Work out the finished part from the listing and answer in its coordinate system (mm). Face numbers are marked on the shaded views. A direction names the side the tool comes from. Coordinates: 2 decimals unless noted, no trailing zeros. Order: outer loops, then holes, each group sorted by start corner. A loop starts at its lowest first (then second) coordinate and runs counter-clockwise, first axis right, second up. Notation, with made-up numbers: M 83.5,79 L 131.5,79 A21 ccw 131.5,106 Z; hole C 33.5,56.5 d3. An arc over 180 degrees is marked long. Answer in a Markdown table with one row per item. Add a question column.
Item 1: Which of the six approach directions +Z, -Z, +X, -X, +Y, -Y give full straight-line access (tool end or side, diameter ignored) to the marked faces 1, 2 and 3?
Item 2: The part is cut by section A-A (y = 55). Write down the section's boundary in (x, z), then the cut area to 3 significant figures.
Item 3: Consider line 1 (Y direction, x = -0.25, z = -1.5); line 2 (Y direction, x = -0.25, z = -4); line 3 (X direction, y = 31.5, z = -8). Determine where each line is inside the solid, lowest interval first. Write a range as from..to.
Item 4: Flat-ended cylindrical pins translate along their axes: pin 1 Ø4 at (x, z) = (1, -6.5) entering from +Y; pin 2 Ø1.7 at (y, z) = (16, -4) entering from +X; pin 3 Ø1.5 at (x, y) = (6, -31.5) entering from +Z. Find the tip coordinate at first contact, or state that the pin passes through.
Item 5: The part is cut by section B-B (z = -2). State how many separate pieces and enclosed holes the cut face has, then the cut area to 3 significant figures.
Item 6: The part is cut by section C-C (y = -76). Write down the section's boundary in (x, z), then the cut area to 3 significant figures.
Item 7: The mould has two halves that part along X. Classify the marked faces 4, 5 and 6: released by +X, released by -X, zero draft, split by the parting line, or undercut.
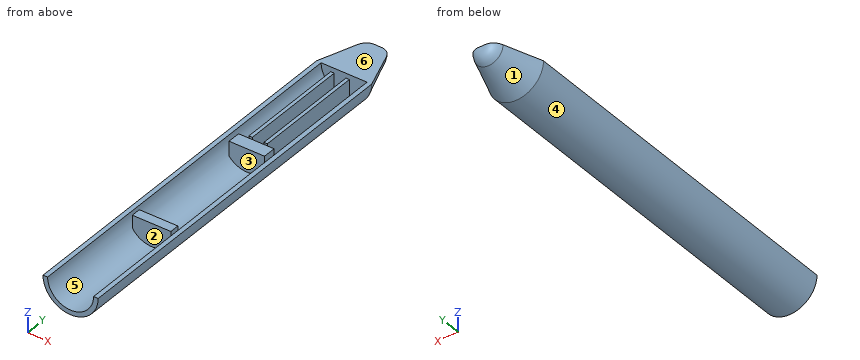
from build123d import *

# Parameters (mm, degrees)
SKETCH2_W                = 2
SKETCH2_H                = 162.039928857
BOSS_EXTRUDE1_REACH      = 94.669
BOSS_EXTRUDE1_END_RADIUS = 10
SKETCH4_W                = 15.457813272
SKETCH4_H                = 5.65259454
SKETCH4_W_2              = 16.763190872
SKETCH4_H_2              = 4.156828513
SKETCH4_W_3              = 1.5
SKETCH4_H_3              = 48.554461885
BOSS_EXTRUDE2_REACH      = 104.169
BOSS_EXTRUDE2_START      = -9.5
SKETCH4_4_W              = 5.08
SKETCH4_4_H              = 48.554461885
SKETCH5_W                = 72.783621468
SKETCH5_H                = 192.84631039
CUT_EXTRUDE1_DEPTH       = 93.66850023


with BuildPart() as part:
    # Sketch1 → Revolve1 (revolve)
    with BuildSketch(Plane.XY, mode=Mode.PRIVATE) as revolve1_sk:
        with BuildLine():
            Line((6.354000149, 87.279039692), (12, 71))
            Line((12, 71), (0, 71))
            Line((0, 71), (0, 91))
            add(Edge.make_bspline(
                [(0, 91), (4.668589185, 91.723642341), (6.354000149, 87.279039692)],
                knots=[0, 0, 0, 1, 1, 1], degree=2))
        make_face()
    revolve(revolve1_sk.sketch.rotate(Axis((0, 91, 0), (0, -1, 0)), 180), axis=Axis((0, 91, 0), (0, -1, 0)))

    # Sketch2 → Revolve2 (revolve)
    with BuildSketch(Plane.XY, mode=Mode.PRIVATE) as revolve2_sk:
        with Locations((11, -10.019964429)):
            Rectangle(SKETCH2_W, SKETCH2_H)
    revolve(revolve2_sk.sketch.rotate(Axis((0, 91, 0), (0, -1, 0)), 180), axis=Axis((0, 91, 0), (0, -1, 0)))

    # Boss-Extrude1: up to this cylinder (the profile starts inside it)
    boss_extrude1_end = Plane(origin=(0, 1.68519, 0), z_dir=(0, 1, 0)) * Cylinder(BOSS_EXTRUDE1_END_RADIUS, 295.657228, mode=Mode.PRIVATE)
    # Sketch4 → Boss-Extrude1 (add, up to the surface)
    with BuildSketch(Plane.XY, mode=Mode.PRIVATE) as boss_extrude1_sk1:
        with Locations((0, 16.17370273)):
            Rectangle(SKETCH4_W, SKETCH4_H)
    boss_extrude1_tool1 = extrude(boss_extrude1_sk1.sketch, amount=-BOSS_EXTRUDE1_REACH, mode=Mode.PRIVATE) & boss_extrude1_end
    add(boss_extrude1_tool1.solids().sort_by_distance((0, 16.173703, 0))[0])
    # Sketch4 → Boss-Extrude1 (add, up to the surface)
    with BuildSketch(Plane.XY, mode=Mode.PRIVATE) as boss_extrude1_sk2:
        with Locations((0, -40.974423961)):
            Rectangle(SKETCH4_W_2, SKETCH4_H_2)
    boss_extrude1_tool2 = extrude(boss_extrude1_sk2.sketch, amount=-BOSS_EXTRUDE1_REACH, mode=Mode.PRIVATE) & boss_extrude1_end
    add(boss_extrude1_tool2.solids().sort_by_distance((0, -40.974424, 0))[0])
    # Sketch4 → Boss-Extrude1 (add, up to the surface)
    with BuildSketch(Plane.XY, mode=Mode.PRIVATE) as boss_extrude1_sk3:
        with Locations((3.29, 44.344804049)):
            Rectangle(SKETCH4_W_3, SKETCH4_H_3)
    boss_extrude1_tool3 = extrude(boss_extrude1_sk3.sketch, amount=-BOSS_EXTRUDE1_REACH, mode=Mode.PRIVATE) & boss_extrude1_end
    add(boss_extrude1_tool3.solids().sort_by_distance((3.29, 44.344804, 0))[0])
    # Sketch4 → Boss-Extrude1 (add, up to the surface)
    with BuildSketch(Plane.XY, mode=Mode.PRIVATE) as boss_extrude1_sk4:
        with Locations((-3.29, 44.344804049)):
            Rectangle(SKETCH4_W_3, SKETCH4_H_3)
    boss_extrude1_tool4 = extrude(boss_extrude1_sk4.sketch, amount=-BOSS_EXTRUDE1_REACH, mode=Mode.PRIVATE) & boss_extrude1_end
    add(boss_extrude1_tool4.solids().sort_by_distance((-3.29, 44.344804, 0))[0])

    # Sketch4<4> → Boss-Extrude2 (add, up to next)
    with BuildSketch(Plane.XY.offset(BOSS_EXTRUDE2_START), mode=Mode.PRIVATE) as boss_extrude2_sk1:
        with Locations((0, 44.344804049)):
            Rectangle(SKETCH4_4_W, SKETCH4_4_H)
    boss_extrude2_tool1 = extrude(boss_extrude2_sk1.sketch, amount=-BOSS_EXTRUDE2_REACH, mode=Mode.PRIVATE) - part.part
    add(boss_extrude2_tool1.solids().sort_by_distance((0, 44.344804, -9.5))[0])

    # Sketch5 → Cut-Extrude1 (cut, through all)
    with BuildSketch(Plane.XY):
        Rectangle(SKETCH5_W, SKETCH5_H)
    extrude(amount=CUT_EXTRUDE1_DEPTH, mode=Mode.SUBTRACT)


solid = part.part
Reply:
| question | item | result |
|---|---|---|
| 1 | face 1 | -Z, +Y |
| 1 | face 2 | +Z, -Y |
| 1 | face 3 | +Z |
| 2 | outline | M -12,0 A12 ccw 12,0 L 10,0 A10 cw 4.04,-9.15 L 4.04,0 L 2.54,0 L 2.54,-9.5 L -2.54,-9.5 L -2.54,0 L -4.04,0 L -4.04,-9.15 A10 cw -10,0 Z |
| 2 | area | 99.4 mm2 |
| 3 | line 1 | y = -43.05..-38.9, 13.35..19, 71..91.1 |
| 3 | line 2 | y = -43.05..-38.9, 13.35..19, 71..90.38 |
| 3 | line 3 | x = -8.94..-6, -4.04..-2.54, 2.54..4.04, 6..8.94 |
| 4 | pin 1 | stops at y = 89.97 |
| 4 | pin 2 | stops at x = 11.58 |
| 4 | pin 3 | stops at z = -7.38 |
| 5 | separate pieces | 5 |
| 5 | enclosed holes | 0 |
| 5 | area | 1,290 mm2 |
| 6 | outline | M -12,0 A12 ccw 12,0 L 10,0 A10 cw -10,0 Z |
| 6 | area | 69.1 mm2 |
| 7 | face 4 | split by the parting line |
| 7 | face 5 | undercut |
| 7 | face 6 | zero draft |
